Source: CAD feature listing. Evaluate the final solid. Frame: model axes, mm. A direction names the side the tool comes from. Give positions to 0.01 mm unless a question says otherwise; leave off trailing zeros. Loops run counter-clockwise (first coordinate to the right, second up) from the corner with the lowest first, then second, coordinate; pieces in that order, holes last. Notation, with made-up numbers: M -16.75,0.25 L 18.25,0.25 A19 cw 18.25,23.25 Z; hole C -31,22 d3. An arc over 180 degrees is marked long. Write item = value, one per line.
from build123d import *

# Parameters (mm, degrees)
F0_W   = 44.45
F0_H   = 44.45
F0_W_2 = 40.2336
F0_H_2 = 40.2336
F4_W   = 44.45
F4_H   = 44.45


with BuildPart() as f2:
    # F2: sweep along a path in F1
    with BuildLine(Plane.XZ) as f2_path:
        Line((-26.4134310049, 0), (-26.4134310049, -152.4))
        Line((-26.4134310049, -152.4), (90.3317421264, -250.3608317162))
        Line((90.3317421264, -250.3608317162), (572.9317421264, -250.3608317162))
        Line((572.9317421264, -250.3608317162), (700.2069564241, -166.5349417689))
        Line((700.2069564241, -166.5349417689), (700.2069564241, -64.9349417689))
    # F0 (on Top) → F2 (sweep)
    with BuildSketch(Plane.XY):
        with Locations((22.225, 22.225)):
            Rectangle(F0_W, F0_H)
        with Locations((22.225, 22.225)):
            Rectangle(F0_W_2, F0_H_2, mode=Mode.SUBTRACT)
    sweep(path=f2_path.line, transition=Transition.RIGHT)

    # F3: F2 across plane


with BuildPart() as f2_1:
    add(f2.part)
    add(f2.part.mirror(Plane.XY))

    # F6: sweep along a path in F5
    with BuildLine(Plane(origin=(0, 0, -223.9474007113), x_dir=(1, 0, 0), z_dir=(0, 0, -1))) as f6_path:
        Line((310.839508958, 21.8996291945), (310.839508958, 210.8011354046))
    # F4 (on face) → F6 (sweep)
    with BuildSketch(Plane.XZ):
        with Locations((311.6830310474, -201.7224007113)):
            Rectangle(F4_W, F4_H)
    sweep(path=f6_path.line)

    # F7: F2 across plane


with BuildPart() as f2_2:
    add(f2_1.part)
    add(f2_1.part.mirror(Plane.XY))


solid = f2_2.part
1. Material intervals for probe 1 along X at (y, z) = (19.5, -73); probe 2 along Z at (x, y) = (122.5, 31); probe 3 along X at (y, z) = (3, -50), sorted ascending. Write a range as from..to.
Derived:
probe_1 = 0..2.11, 42.34..44.45, 629.34..631.45, 671.69..673.79
probe_2 = -223.95..-221.84, -181.61..-179.5, 179.5..181.61, 221.84..223.95
probe_3 = 0..2.11, 42.34..44.45
2. Cut plane A-A, the plane z = -89.5. Return the cut outline in (x, y), then the cut area to 3 significant figures.
Derived:
outline = M 0,0 L 44.45,0 L 44.45,44.45 L 0,44.45 Z; M 629.34,0 L 673.79,0 L 673.79,44.45 L 629.34,44.45 Z; hole M 2.11,2.11 L 42.34,2.11 L 42.34,42.34 L 2.11,42.34 Z; hole M 631.45,2.11 L 671.69,2.11 L 671.69,42.34 L 631.45,42.34 Z
area = 714 mm²
3. Cut plane B-B, the plane x = 318. Return the cut outline in (y, z), then the cut area to 3 significant figures.
Derived:
outline = M -188.9,-223.95 L 44.45,-223.95 L 44.45,-179.5 L -188.9,-179.5 Z; M -188.9,179.5 L 44.45,179.5 L 44.45,223.95 L -188.9,223.95 Z; hole M 2.11,-221.84 L 42.34,-221.84 L 42.34,-181.61 L 2.11,-181.61 Z; hole M 2.11,181.61 L 42.34,181.61 L 42.34,221.84 L 2.11,221.84 Z
area = 17,500 mm²
4. Cut plane D-D, the plane z = -37.5. Return the cut outline in (x, y), then the cut area to 3 significant figures.
Derived:
outline = M 0,0 L 44.45,0 L 44.45,44.45 L 0,44.45 Z; hole M 2.11,2.11 L 42.34,2.11 L 42.34,42.34 L 2.11,42.34 Z
area = 357 mm²
5. Reachability of faces 1 (the flat face through (629.344, 22, -96)), 2 (the flat face through (620.2, 22.5, -187.6)), 3 (the flat face through (592.442, 22.507, 155.183)), 4 (the flat face through (653, 1, 64.935)), 5 (the flat face through (333.908, -96, -202)) from +Z, -Z, +X, -X, +Y, -Y: full face, straight path, thin tool, end or side. Return the list, or none.
Derived:
face_1 = +Y, -Y
face_2 = -Z, +X, +Y, -Y
face_3 = none
face_4 = +X, +Y, -Y
face_5 = +Z, -Z, +X, -Y
6. Cut plane C-C, the plane y = -104.5. Return the cut outline in (x, z), then the cut area to 3 significant figures.
Derived:
outline = M 289.46,-223.95 L 333.91,-223.95 L 333.91,-179.5 L 289.46,-179.5 Z; M 289.46,179.5 L 333.91,179.5 L 333.91,223.95 L 289.46,223.95 Z
area = 3,950 mm²
7. Pull-direction query (X, two-part tool) for faces 6 (the flat face through (289.458, -96, -201)), 7 (the flat face through (673.794, 23, -108)), 8 (the flat face through (44.45, 22, 2)); classes: +X half, -X half, draft (parallel to the pull), parting line (faces both ways), or undercut.
Derived:
face_6 = -X half
face_7 = +X half
face_8 = undercut
8. First-contact query: pin 1 Ø13.5 at (y, z) = (-92.5, -198) entering from -X; pin 2 Ø20 at (y, z) = (27, -3.5) entering from +X. Flat tips, straight axial feed; report the tip coordinate or a pass-through.
Derived:
pin_1 = 289.46
pin_2 = 44.45
